Input: part model. Units: mm. Frame: model coordinates. Coordinates: 2 decimals unless noted, no trailing zeros. One line per item, written item: value.
```python
from build123d import *

# Parameters (mm, degrees)
F0_W     = 178
F0_H     = 132
F0_R     = 1.6
F0_R_2   = 1.85
F0_R_3   = 4
F1_DEPTH = 25


with BuildPart() as f1:
    # F0 (on Front) → F1 (new body)
    with BuildSketch(Plane.XZ):
        with Locations((0, -66)):
            Rectangle(F0_W, F0_H)
        with Locations((-40, -127)):
            Circle(F0_R, mode=Mode.SUBTRACT)
        with Locations((-78.656854, -85.656854)):
            Circle(F0_R_2, mode=Mode.SUBTRACT)
        with Locations((-73, -88)):
            Circle(F0_R_2, mode=Mode.SUBTRACT)
        with Locations((-67.343146, -85.656854)):
            Circle(F0_R_2, mode=Mode.SUBTRACT)
        with Locations((-81, -80)):
            Circle(F0_R_2, mode=Mode.SUBTRACT)
        with Locations((-78.656854, -74.343146)):
            Circle(F0_R_2, mode=Mode.SUBTRACT)
        with Locations((-73, -80)):
            Circle(F0_R_3, mode=Mode.SUBTRACT)
        with Locations((-67.343146, -74.343146)):
            Circle(F0_R_2, mode=Mode.SUBTRACT)
        with Locations((-73, -72)):
            Circle(F0_R_2, mode=Mode.SUBTRACT)
        with Locations((-65, -80)):
            Circle(F0_R_2, mode=Mode.SUBTRACT)
        with Locations((-40, -71)):
            Circle(F0_R, mode=Mode.SUBTRACT)
        with Locations((39, -127)):
            Circle(F0_R, mode=Mode.SUBTRACT)
        with Locations((39, -71)):
            Circle(F0_R, mode=Mode.SUBTRACT)
        with Locations((65.343146, -85.656854)):
            Circle(F0_R_2, mode=Mode.SUBTRACT)
        with Locations((71, -88)):
            Circle(F0_R_2, mode=Mode.SUBTRACT)
        with Locations((76.656854, -85.656854)):
            Circle(F0_R_2, mode=Mode.SUBTRACT)
        with Locations((63, -80)):
            Circle(F0_R_2, mode=Mode.SUBTRACT)
        with Locations((65.343146, -74.343146)):
            Circle(F0_R_2, mode=Mode.SUBTRACT)
        with Locations((71, -80)):
            Circle(F0_R_3, mode=Mode.SUBTRACT)
        with Locations((76.656854, -74.343146)):
            Circle(F0_R_2, mode=Mode.SUBTRACT)
        with Locations((79, -80)):
            Circle(F0_R_2, mode=Mode.SUBTRACT)
        with Locations((71, -72)):
            Circle(F0_R_2, mode=Mode.SUBTRACT)
        with Locations((-40, -60)):
            Circle(F0_R, mode=Mode.SUBTRACT)
        with Locations((-78.656854, -21.656854)):
            Circle(F0_R_2, mode=Mode.SUBTRACT)
        with Locations((-73, -24)):
            Circle(F0_R_2, mode=Mode.SUBTRACT)
        with Locations((-67.343146, -21.656854)):
            Circle(F0_R_2, mode=Mode.SUBTRACT)
        with Locations((-81, -16)):
            Circle(F0_R_2, mode=Mode.SUBTRACT)
        with Locations((-78.656854, -10.343146)):
            Circle(F0_R_2, mode=Mode.SUBTRACT)
        with Locations((-73, -16)):
            Circle(F0_R_3, mode=Mode.SUBTRACT)
        with Locations((-67.343146, -10.343146)):
            Circle(F0_R_2, mode=Mode.SUBTRACT)
        with Locations((-73, -8)):
            Circle(F0_R_2, mode=Mode.SUBTRACT)
        with Locations((-65, -16)):
            Circle(F0_R_2, mode=Mode.SUBTRACT)
        with Locations((-40, -4)):
            Circle(F0_R, mode=Mode.SUBTRACT)
        with Locations((39, -60)):
            Circle(F0_R, mode=Mode.SUBTRACT)
        with Locations((39, -4)):
            Circle(F0_R, mode=Mode.SUBTRACT)
        with Locations((65.343146, -21.656854)):
            Circle(F0_R_2, mode=Mode.SUBTRACT)
        with Locations((71, -24)):
            Circle(F0_R_2, mode=Mode.SUBTRACT)
        with Locations((76.656854, -21.656854)):
            Circle(F0_R_2, mode=Mode.SUBTRACT)
        with Locations((63, -16)):
            Circle(F0_R_2, mode=Mode.SUBTRACT)
        with Locations((65.343146, -10.343146)):
            Circle(F0_R_2, mode=Mode.SUBTRACT)
        with Locations((71, -16)):
            Circle(F0_R_3, mode=Mode.SUBTRACT)
        with Locations((76.656854, -10.343146)):
            Circle(F0_R_2, mode=Mode.SUBTRACT)
        with Locations((79, -16)):
            Circle(F0_R_2, mode=Mode.SUBTRACT)
        with Locations((71, -8)):
            Circle(F0_R_2, mode=Mode.SUBTRACT)
    extrude(amount=F1_DEPTH)


solid = f1.part
```
(1) Ray query, line 1 (Z direction, x = -67, y = -10.75); line 2 (Z direction, x = -81, y = -17); line 3 (Z direction, x = -40, y = -12.5). Return the intervals inside material, ascending. Write a range as from..to.
Data:
line 1: z = -132..-87.47, -83.84..-76.16, -72.53..-23.47, -19.84..-12.16, -8.53..0
line 2: z = -132..-81.85, -78.15..-17.85, -14.15..0
line 3: z = -132..-128.6, -125.4..-72.6, -69.4..-61.6, -58.4..-5.6, -2.4..0
(2) Cut plane A-A on y = -20. Give the number of separate pieces and of enclosed holes in the cut face, plus the area to 3 significant figures.
Data:
separate pieces: 1
enclosed holes: 44
area: 22,900 mm2
(3) First-contact query: pin 1 (10 mm diameter, centred on x = -13.5, z = -80, fed in from +Y). Flat tip, straight axial feed; report the tip coordinate or a pass-through.
Data:
pin 1: stops at y = 0
(4) Draft query along Z for faces 1 (the cylindrical face through (70.599, -12.325, -73.806)), 2 (the flat face through (-1, 0, -65)). Return one class per face: released by +Z, released by -Z, zero draft, split by the parting line, or undercut.
Data:
face 1: undercut
face 2: zero draft
